```python
from build123d import *

# Parameters (mm, degrees)
SKETCH1_W           = 20.5
SKETCH1_H           = 21.55
BOSS_EXTRUDE1_DEPTH = 43.2
FILLET1_R           = 3.2
BOSS_EXTRUDE2_DEPTH = 31.24
CUT_EXTRUDE1_DEPTH  = 10
SKETCH4_W           = 7.87
SKETCH4_H           = 23.5
BOSS_EXTRUDE3_DEPTH = 8
CUT_EXTRUDE2_REACH  = 17.535
SKETCH5_R           = 2.325
SKETCH7_R           = 3.075
CUT_EXTRUDE3_DEPTH  = 0.5
SKETCH8_R           = 3.075
CUT_EXTRUDE5_DEPTH  = 0.5
FILLET2_R           = 4
SKETCH9_W           = 12.28
SKETCH9_H           = 14.55
CUT_EXTRUDE6_DEPTH  = 15
FILLET3_R           = 1


with BuildPart() as part:
    # Sketch1 → Boss-Extrude1 (new body)
    with BuildSketch(Plane.XY):
        with Locations((10.25, 10.775)):
            Rectangle(SKETCH1_W, SKETCH1_H)
    extrude(amount=BOSS_EXTRUDE1_DEPTH)

    # Fillet1
    fillet1_edges = [part.edges().sort_by_distance(p)[0] for p in [
        (20.5, 10.775, 43.2),
        (10.25, 21.55, 43.2),
        (0, 10.775, 43.2),
        (10.25, 0, 43.2),
        (0, 21.55, 21.6),
        (20.5, 21.55, 21.6),
        (20.5, 0, 21.6),
        (0, 0, 21.6),
    ]]
    fillet(fillet1_edges, radius=FILLET1_R)

    # Sketch2 → Boss-Extrude2 (add)
    with BuildSketch(Plane(origin=(0, 0, 5.44), x_dir=(-1, 0, 0), z_dir=(0, 0, -1))):
        with BuildLine():
            Line((-20.5, 10.775), (-21.85, 10.775))
            Line((-21.85, 10.775), (-21.85, 19.7))
            ThreePointArc((-21.85, 19.7), (-20.9127417, 21.9627417), (-18.65, 22.9))
            Line((-18.65, 22.9), (-1.85, 22.9))
            ThreePointArc((-1.85, 22.9), (0.4127417, 21.9627417), (1.35, 19.7))
            Line((1.35, 19.7), (1.35, 10.775))
            Line((1.35, 10.775), (0, 10.775))
            Line((0, 10.775), (0, 18.35))
            ThreePointArc((0, 18.35), (-0.9372583, 20.6127417), (-3.2, 21.55))
            Line((-3.2, 21.55), (-17.3, 21.55))
            ThreePointArc((-17.3, 21.55), (-19.5627417, 20.6127417), (-20.5, 18.35))
            Line((-20.5, 18.35), (-20.5, 10.775))
        make_face()
    extrude(amount=-BOSS_EXTRUDE2_DEPTH)

    # Sketch3 → Cut-Extrude1 (cut)
    with BuildSketch(Plane.XY.offset(43.2)):
        with BuildLine():
            Line((15.19568246, 11.51), (18.515, 11.51))
            ThreePointArc((18.515, 11.51), (19.25, 10.775), (18.515, 10.04))
            Line((18.515, 10.04), (15.19568246, 10.04))
            ThreePointArc((15.19568246, 10.04), (13.785533906, 7.239466094), (10.985, 5.82931754))
            Line((10.985, 5.82931754), (10.985, 2.51))
            ThreePointArc((10.985, 2.51), (10.25, 1.775), (9.515, 2.51))
            Line((9.515, 2.51), (9.515, 5.82931754))
            ThreePointArc((9.515, 5.82931754), (6.714466094, 7.239466094), (5.30431754, 10.04))
            Line((5.30431754, 10.04), (1.985, 10.04))
            ThreePointArc((1.985, 10.04), (1.25, 10.775), (1.985, 11.51))
            Line((1.985, 11.51), (5.30431754, 11.51))
            ThreePointArc((5.30431754, 11.51), (6.714466094, 14.310533906), (9.515, 15.72068246))
            Line((9.515, 15.72068246), (9.515, 19.04))
            ThreePointArc((9.515, 19.04), (10.25, 19.775), (10.985, 19.04))
            Line((10.985, 19.04), (10.985, 15.72068246))
            ThreePointArc((10.985, 15.72068246), (13.785533906, 14.310533906), (15.19568246, 11.51))
        make_face()
    extrude(amount=-CUT_EXTRUDE1_DEPTH, mode=Mode.SUBTRACT)

    # Sketch4 → Boss-Extrude3 (add)
    with BuildSketch(Plane.XZ):
        with Locations((10.25, 11.75)):
            Rectangle(SKETCH4_W, SKETCH4_H)
    extrude(amount=BOSS_EXTRUDE3_DEPTH)

    # Sketch5 → Cut-Extrude2 (cut, up to next)
    with BuildSketch(Plane(origin=(14.185, 0, 0), x_dir=(0, 0, -1), z_dir=(1, 0, 0)), mode=Mode.PRIVATE) as cut_extrude2_sk1:
        with Locations((-19.75, -4)):
            Circle(SKETCH5_R)
    cut_extrude2_tool1 = extrude(cut_extrude2_sk1.sketch, amount=-CUT_EXTRUDE2_REACH, mode=Mode.PRIVATE) & part.part
    add(cut_extrude2_tool1.solids().sort_by_distance((14.185, -4, 19.75))[0], mode=Mode.SUBTRACT)
    # Sketch5 → Cut-Extrude2 (cut, up to next)
    with BuildSketch(Plane(origin=(14.185, 0, 0), x_dir=(0, 0, -1), z_dir=(1, 0, 0)), mode=Mode.PRIVATE) as cut_extrude2_sk2:
        with Locations((-11.75, -4)):
            Circle(SKETCH5_R)
    cut_extrude2_tool2 = extrude(cut_extrude2_sk2.sketch, amount=-CUT_EXTRUDE2_REACH, mode=Mode.PRIVATE) & part.part
    add(cut_extrude2_tool2.solids().sort_by_distance((14.185, -4, 11.75))[0], mode=Mode.SUBTRACT)
    # Sketch5 → Cut-Extrude2 (cut, up to next)
    with BuildSketch(Plane(origin=(14.185, 0, 0), x_dir=(0, 0, -1), z_dir=(1, 0, 0)), mode=Mode.PRIVATE) as cut_extrude2_sk3:
        with Locations((-3.75, -4)):
            Circle(SKETCH5_R)
    cut_extrude2_tool3 = extrude(cut_extrude2_sk3.sketch, amount=-CUT_EXTRUDE2_REACH, mode=Mode.PRIVATE) & part.part
    add(cut_extrude2_tool3.solids().sort_by_distance((14.185, -4, 3.75))[0], mode=Mode.SUBTRACT)

    # Sketch7 → Cut-Extrude3 (cut)
    with BuildSketch(Plane(origin=(14.185, 0, 0), x_dir=(0, 0, -1), z_dir=(1, 0, 0))):
        with Locations((-19.75, -4)):
            Circle(SKETCH7_R)
        with Locations((-11.75, -4)):
            Circle(SKETCH7_R)
        with Locations((-3.75, -4)):
            Circle(SKETCH7_R)
    extrude(amount=-CUT_EXTRUDE3_DEPTH, mode=Mode.SUBTRACT)

    # Sketch8 → Cut-Extrude5 (cut)
    with BuildSketch(Plane.ZY.offset(-6.315)):
        with Locations((3.75, -4)):
            Circle(SKETCH8_R)
        with Locations((11.75, -4)):
            Circle(SKETCH8_R)
        with Locations((19.75, -4)):
            Circle(SKETCH8_R)
    extrude(amount=-CUT_EXTRUDE5_DEPTH, mode=Mode.SUBTRACT)

    # Fillet2
    fillet2_edges = [part.edges().sort_by_distance(p)[0] for p in [
        (10.25, -8, 0),
        (10.25, -8, 23.5),
    ]]
    fillet(fillet2_edges, radius=FILLET2_R)

    # Sketch9 → Cut-Extrude6 (cut)
    with BuildSketch(Plane(origin=(0, 0, 0), x_dir=(-1, 0, 0), z_dir=(0, 0, -1))):
        with Locations((-10.25, 7.775)):
            Rectangle(SKETCH9_W, SKETCH9_H)
    extrude(amount=-CUT_EXTRUDE6_DEPTH, mode=Mode.SUBTRACT)

    # Fillet3
    fillet3_edges = [part.edges().sort_by_distance(p)[0] for p in [
        (16.39, 0.5, 7.5),
        (4.11, 0.5, 7.5),
    ]]
    fillet(fillet3_edges, radius=FILLET3_R)


solid = part.part
```
Geometry check sheet. Reference: the model listing, model coordinates, mm. A direction names the side the tool comes from. Give positions to 0.01 mm unless a question says otherwise; leave off trailing zeros. Order: outer loops, then holes, each group sorted by start corner. A loop starts at its lowest first (then second) coordinate and runs counter-clockwise, first axis right, second up.
1. Section check B-B, the plane z = 38. Enter the section's corners in (x, y) (3 decimals).
2. Gauge pin test, flat ends, axial feed: pin 1 Ø8 at (y, z) = (-1, 5) entering from +X; pin 2 Ø5 at (y, z) = (-4, 11.75) entering from -X (3 decimals); pin 3 Ø1.7 at (x, z) = (17, 39) entering from +Y. Record the tip position at first contact, or that the pin passes through.
3. Section check A-A, the plane z = 11.75. Give the number of separate pieces and of enclosed holes in the cut face, and give its area (3 significant figures).
4. Section check C-C, the plane x = 11.75. Enter the section's corners in (y, z) (3 decimals).
5. Access from +Z, -Z, +X, -X, +Y, -Y to the whole of each face (thin tool, end or side, straight path). Record for faces 1 (the face through (10, 15.05, 7)), 2 (the face through (10, 21.55, 38)), 3 (the face through (6.562, -6.728, 5.169)), 4 (the face through (19.587, 20.588, 2.758)).
6. Release check for a two-part mould opening along X. For faces 5 (the face through (6, 16, 43.2)), 6 (the face through (16.105, 0.801, 7.605)), 7 (the face through (0.913, 20.588, 38.363)) record: pulls with the +X half, pulls with the -X half, needs draft (parallel to the pull), parting line crosses it, or undercut.
7. Thickness scan on L1, parallel to Y at x = 6.7, z = 11.75 (3 decimals); L2, parallel to Y at x = 6.55, z = 19.75 (3 decimals); L3, parallel to X at y = 3.5, z = 2.5. Record the ranges inside material, lowest first.
8. Section check D-D, the plane y = 8.5. Enter the section's corners in (x, z), and give its area (3 significant figures).
Values follow:
1. outline: (0, 3.2) arc R3.2 ccw to (3.2, 0) - (17.3, 0) arc R3.2 ccw to (20.5, 3.2) - (20.5, 18.35) arc R3.2 ccw to (17.3, 21.55) - (3.2, 21.55) arc R3.2 ccw to (0, 18.35) - close; hole (1.985, 10.04) - (5.304, 10.04) arc R5 ccw to (9.515, 5.829) - (9.515, 2.51) arc R0.735 ccw to (10.985, 2.51) - (10.985, 5.829) arc R5 ccw to (15.196, 10.04) - (18.515, 10.04) arc R0.735 ccw to (18.515, 11.51) - (15.196, 11.51) arc R5 ccw to (10.985, 15.721) - (10.985, 19.04) arc R0.735 ccw to (9.515, 19.04) - (9.515, 15.721) arc R5 ccw to (5.304, 11.51) - (1.985, 11.51) arc R0.735 ccw to start
2. pin 1: stops at x = 20.49
2. pin 2: stops at x = 6.815
2. pin 3: stops at y = 21.55
3. separate pieces: 2
3. enclosed holes: 1
3. area: 340 mm2
4. outline: (-8, 4) arc R4 ccw to (-4, 0) - (0.5, 0) - (0.5, 15) - (15.05, 15) - (15.05, 0) - (21.55, 0) - (21.55, 5.44) - (22.9, 5.44) - (22.9, 36.68) - (21.55, 36.68) - (21.55, 40) arc R3.2 ccw to (18.35, 43.2) - (15.545, 43.2) - (15.545, 33.2) - (6.005, 33.2) - (6.005, 43.2) - (3.2, 43.2) arc R3.2 ccw to (0, 40) - (0, 23.5) - (-4, 23.5) arc R4 ccw to (-8, 19.5) - close; hole circle Ø4.65 at (-4, 3.75); hole circle Ø4.65 at (-4, 11.75); hole circle Ø4.65 at (-4, 19.75)
5. face 1: -Z
5. face 2: +Z, +X, -X, +Y
5. face 3: -X
5. face 4: -Z, +X, +Y
6. face 5: needs draft
6. face 6: undercut
6. face 7: pulls with the -X half
7. L1: y = -8 to -7.075, -0.925 to 0.5, 15.05 to 22.9
7. L2: y = -7.992 to -7.075, -0.925 to 22.9
7. L3: x = 0 to 4.11, 16.39 to 20.5
8. outline: (0, 0) - (4.11, 0) - (4.11, 15) - (16.39, 15) - (16.39, 0) - (20.5, 0) - (20.5, 40) arc R3.2 ccw to (17.3, 43.2) - (14.7, 43.2) - (14.7, 33.2) - (5.8, 33.2) - (5.8, 43.2) - (3.2, 43.2) arc R3.2 ccw to (0, 40) - close
8. area: 608 mm2
